Geometry check sheet. Reference: drawing and pictorial views, mm from the part's lowest x, y, z. A direction names the side the tool comes from. Give positions to 0.01 mm unless a question says otherwise; leave off trailing zeros. Order: outer loops, then holes, each group sorted by start corner. A loop starts at its lowest first (then second) coordinate and runs counter-clockwise, first axis right, second up.
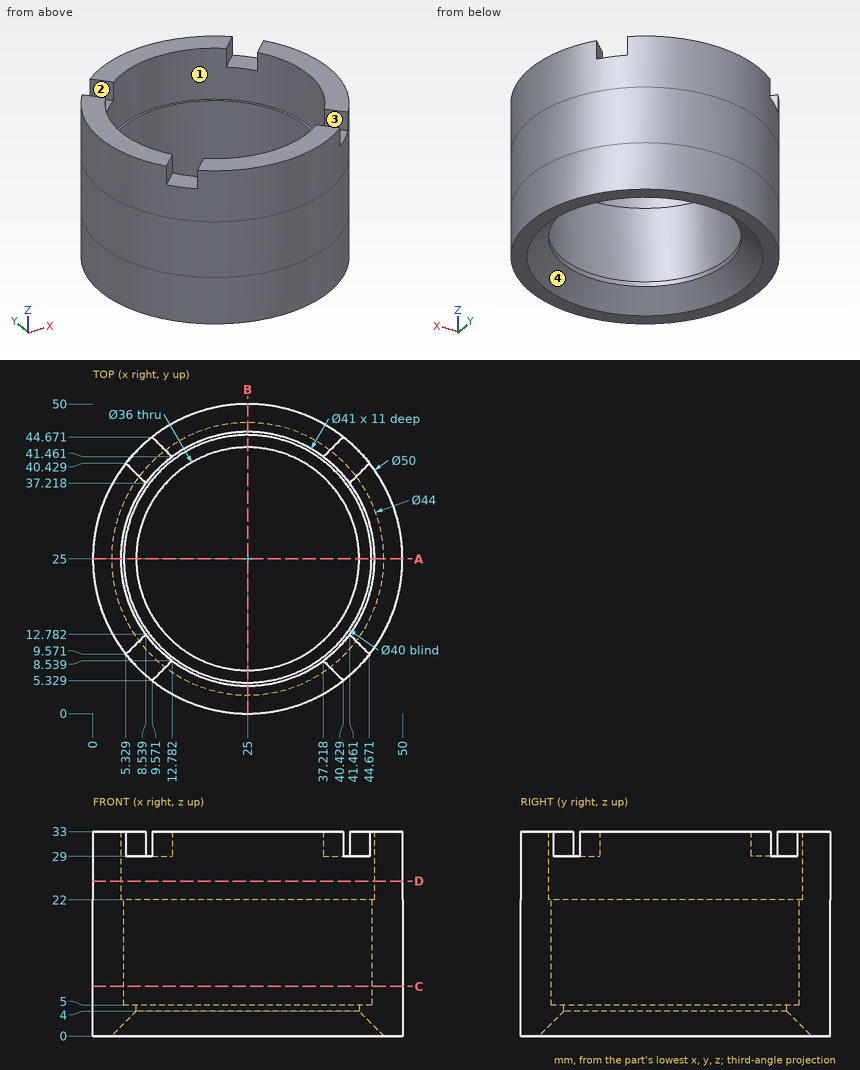
1) Section check A-A, the plane y = 25. Record the cut outline in (x, z).
Recorded:
outline: (0, 0) - (3, 0) - (7, 4) - (7, 5) - (5, 5) - (5, 22) - (4.5, 22) - (4.5, 33) - (0, 33) - close; (43, 4) - (47, 0) - (50, 0) - (50, 33) - (45.5, 33) - (45.5, 22) - (45, 22) - (45, 5) - (43, 5) - close
2) Set-up check for the marked faces 1, 2, 3 and 4: record each of +Z, -Z, +X, -X, +Y, -Y from which the full face is reachable in a straight line by a thin tool's end or side.
Recorded:
face 1: +Z
face 2: +Z, -X
face 3: +Z, -Y
face 4: -Z
3) Depth check by flat-ended pin: pin 1 Ø8 at (x, z) = (30, 10.5) entering from -Y; pin 2 Ø1.5 at (x, z) = (27.5, 13.5) entering from +Y; pin 3 Ø3.5 at (x, y) = (41.5, 10) entering from +Z; pin 4 Ø12 at (x, y) = (27.5, 18.5) entering from +Z. Enter the tip coordinate at first touch or a pass-through.
Recorded:
pin 1: stops at y = 0.02
pin 2: stops at y = 49.94
pin 3: stops at z = 29
pin 4: passes through
4) Section check C-C, the plane z = 8. Record the cut outline in (x, y).
Recorded:
outline: circle Ø50 at (25, 25); hole circle Ø40 at (25, 25)
5) Section check D-D, the plane z = 25. Record the cut outline in (x, y), then the cut area to 3 significant figures.
Recorded:
outline: circle Ø50 at (25, 25); hole circle Ø41 at (25, 25)
area: 643 mm2
6) Material ranges on L1, parallel to Y at x = 25, z = 16; L2, parallel to X at y = 25, z = 26; L3, parallel to Y at x = 25, z = 4.7, recorded low to high.
Recorded:
L1: y = 0 to 5, 45 to 50
L2: x = 0 to 4.5, 45.5 to 50
L3: y = 0 to 7, 43 to 50
